Check sheet for the drawn part. Datum: minimum x, y, z corner. Units: mm. A direction names the side the tool comes from. Coordinates: 2 decimals unless noted, no trailing zeros. Loops run counter-clockwise (first coordinate to the right, second up) from the corner with the lowest first, then second, coordinate; pieces in that order, holes last.
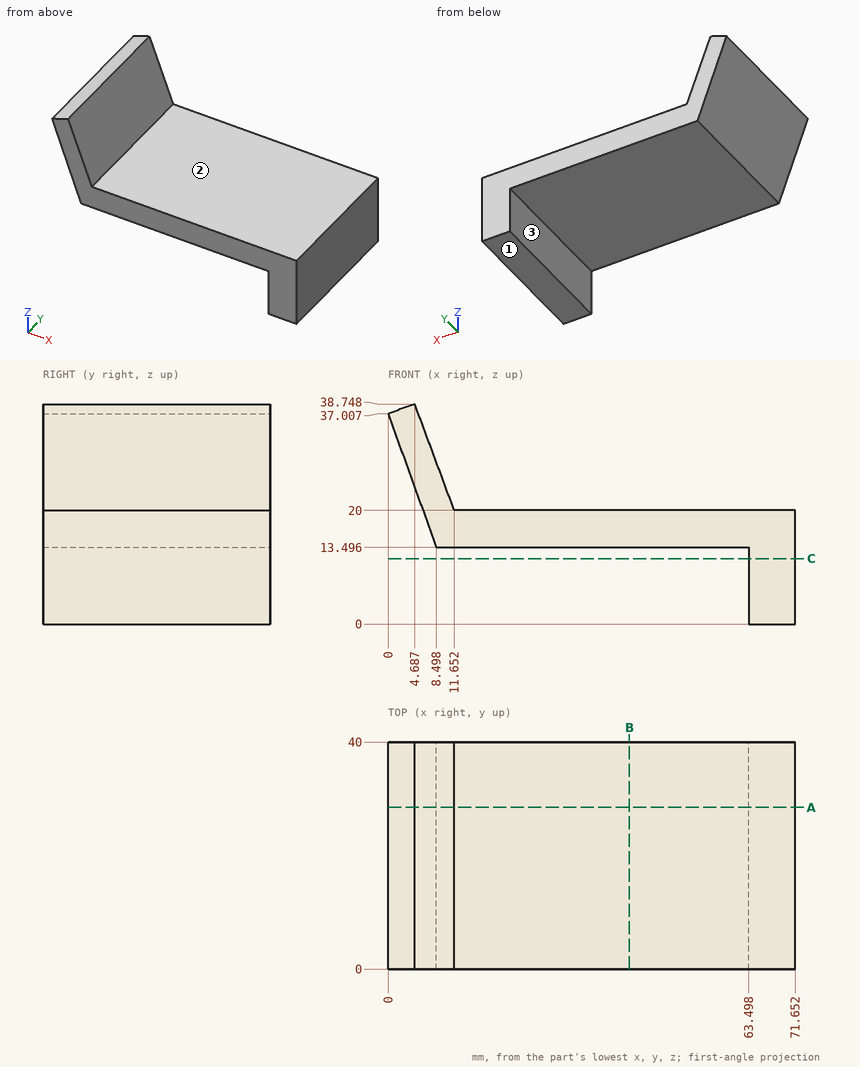
1) Scan lines: line 1 (Z direction, x = 67, y = 20); line 2 (X direction, y = 10, z = 7); line 3 (Z direction, x = 59, y = 20) (1 decimal). Record each from-to range of solid material in increasing order.
Answer sheet:
line 1: z = 0 to 20
line 2: x = 63.5 to 71.65
line 3: z = 13.5 to 20
2) Section check B-B on x = 42.5. Enter the section's corners in (y, z) (1 decimal).
Answer sheet:
outline: (0, 13.5) - (40, 13.5) - (40, 20) - (0, 20) - close
3) Set-up check for the marked faces 1, 2 and 3: record each of +Z, -Z, +X, -X, +Y, -Y from which the full face is reachable in a straight line by a thin tool's end or side.
Answer sheet:
face 1: -Z, +X, -X, +Y, -Y
face 2: +Z, +X, +Y, -Y
face 3: -Z, -X, +Y, -Y
4) Depth check by flat-ended pin: pin 1 (12 mm diameter, centred on x = 33.5, y = 16.5, fed in from -Z); pin 2 (11 mm diameter, centred on y = 26, z = 9.5, fed in from -X) (1 decimal); pin 3 (1.5 mm diameter, centred on x = 28, y = 11.5, fed in from +Z). Enter the tip coordinate at first touch or a pass-through.
Answer sheet:
pin 1: stops at z = 13.5
pin 2: stops at x = 8
pin 3: stops at z = 20
5) Section check A-A on y = 28.5. Enter the section's corners in (x, z) (1 decimal).
Answer sheet:
outline: (0, 37) - (8.5, 13.5) - (63.5, 13.5) - (63.5, 0) - (71.7, 0) - (71.7, 20) - (11.7, 20) - (4.7, 38.7) - close
6) Section check C-C on z = 11.5. Enter the section's corners in (x, y), plus the area to 3 significant figures.
Answer sheet:
outline: (63.5, 0) - (71.65, 0) - (71.65, 40) - (63.5, 40) - close
area: 326 mm2
